Geometry: final body of the model. Coordinates: model frame, mm. A direction names the side the tool comes from. Round coordinates to 2 decimals unless told otherwise and drop trailing zeros. Write each loop counter-clockwise with the first axis right and the second up, starting at its lowest first coordinate (ties: lowest second). Pieces come first, ordered by that corner, then holes. Notation, with made-up numbers: (62.5, -7) -> (111.5, -7) arc R19 cw to (111.5, 4) -> close; hole circle Ø3 at (41.25, 0.25). An arc over 180 degrees is marked (long way). Use one line per item in the form item = value. Start each with the question number.
1. Cut plane D-D, the plane x = 1. Return the cut outline in (y, z), plus the area to 3 significant figures.
2. Pin query (flat end, axial travel): pin 1 Ø3.5 at (x, z) = (48, 0) entering from -Y; pin 2 Ø3 at (x, z) = (15, -0.5) entering from +Y; pin 3 Ø1 at (y, z) = (3.5, 1.5) entering from +X; pin 4 Ø1.5 at (y, z) = (3, 1) entering from -X. Return the tip coordinate at first contact, or that it passes through.
3. Reachability of faces 1 (the face through (20.974, 0.493, 0.672)), 2 (the face through (42, 7, -2)), 3 (the face through (36, 4, -3.1)) from +Z, -Z, +X, -X, +Y, -Y: full face, straight path, thin tool, end or side. Return the list, or none.
4. Cut plane B-B, the plane y = 7.5. State how many separate pieces and enclosed holes the cut face has, plus the area to 3 significant figures.
5. Cut plane A-A, the plane x = 24. Return the cut outline in (y, z).
6. Line query: L1, parallel to Z at x = 28, y = 5; L2, parallel to Y at x = 37.5, z = 1; L3, parallel to Z at x = 39, y = 5. Output: solid intervals per line, ascending.
```python
from build123d import *

# Parameters (mm, degrees)
BOSS_EXTRUDE1_DEPTH = 8
SKETCH5_R           = 3.1
CUT_EXTRUDE1_DEPTH  = 1
SKETCH6_R           = 2.4
CUT_EXTRUDE2_DEPTH  = 53.091266063
CUT_EXTRUDE3_START  = -1
SKETCH8_R           = 3.1
CUT_EXTRUDE3_DEPTH  = 1
LPATTERN3_COUNT     = 7
LPATTERN3_PITCH     = 8
CUT_EXTRUDE4_DEPTH  = 53.235045707
LPATTERN4_COUNT     = 6
LPATTERN4_PITCH     = 8


with BuildPart() as part:
    # Sketch3 → Boss-Extrude1 (new body)
    with BuildSketch(Plane(origin=(0, 0, 0), x_dir=(1, 0, 0), z_dir=(0, 1, 0))):
        with BuildLine():
            Line((0, 3.5), (48, 3.5))
            ThreePointArc((48, 3.5), (51.5, 0), (48, -3.5))
            Line((48, -3.5), (0, -3.5))
            ThreePointArc((0, -3.5), (-3.5, 0), (0, 3.5))
        make_face()
    extrude(amount=BOSS_EXTRUDE1_DEPTH)

    # Sketch5 → Cut-Extrude1 (cut)
    with BuildSketch(Plane(origin=(0, 0, 0), x_dir=(-1, 0, 0), z_dir=(0, -1, 0))):
        with Locations(Location((0, 0, 0), (0, 0, 90))):
            Circle(SKETCH5_R)
    cut_extrude1 = extrude(amount=-CUT_EXTRUDE1_DEPTH, mode=Mode.SUBTRACT)

    # Sketch6 → Cut-Extrude2 (cut, symmetric)
    with BuildSketch(Plane(origin=(0, 1, 0), x_dir=(-1, 0, 0), z_dir=(0, -1, 0))):
        with Locations(Location((0, 0, 0), (0, 0, 90))):
            Circle(SKETCH6_R)
    cut_extrude2 = extrude(amount=CUT_EXTRUDE2_DEPTH, both=True, mode=Mode.SUBTRACT)

    # Sketch8 → Cut-Extrude3 (cut)
    with BuildSketch(Plane(origin=(0, 8, 0), x_dir=(1, 0, 0), z_dir=(0, 1, 0)).offset(CUT_EXTRUDE3_START)):
        with Locations(Location((0, 0, 0), (0, 0, 90))):
            Circle(SKETCH8_R)
    cut_extrude3 = extrude(amount=CUT_EXTRUDE3_DEPTH, mode=Mode.SUBTRACT)

    # LPattern3: Cut-Extrude1, Cut-Extrude2, Cut-Extrude3 ×7
    with Locations(*[(i * LPATTERN3_PITCH, 0, 0) for i in range(1, LPATTERN3_COUNT)]):
        add(cut_extrude1, mode=Mode.SUBTRACT)
        add(cut_extrude2, mode=Mode.SUBTRACT)
        add(cut_extrude3, mode=Mode.SUBTRACT)

    # Sketch9 → Cut-Extrude4 (cut, symmetric)
    with BuildSketch(Plane(origin=(0, 8, 0), x_dir=(1, 0, 0), z_dir=(0, 1, 0))):
        with BuildLine():
            Line((2.814249456, 3.1), (5.185750544, 3.1))
            ThreePointArc((5.185750544, 3.1), (5.553697029, 2.856892908), (5.474391514, 2.423076923))
            ThreePointArc((5.474391514, 2.423076923), (4.5, 0), (5.474391514, -2.423076923))
            ThreePointArc((5.474391514, -2.423076923), (5.553697029, -2.856892908), (5.185750544, -3.1))
            Line((5.185750544, -3.1), (2.814249456, -3.1))
            ThreePointArc((2.814249456, -3.1), (2.446302971, -2.856892908), (2.525608486, -2.423076923))
            ThreePointArc((2.525608486, -2.423076923), (3.5, 0), (2.525608486, 2.423076923))
            ThreePointArc((2.525608486, 2.423076923), (2.446302971, 2.856892908), (2.814249456, 3.1))
        make_face()
    cut_extrude4 = extrude(amount=CUT_EXTRUDE4_DEPTH, both=True, mode=Mode.SUBTRACT)

    # LPattern4: Cut-Extrude4 ×6
    with Locations(*[(i * LPATTERN4_PITCH, 0, 0) for i in range(1, LPATTERN4_COUNT)]):
        add(cut_extrude4, mode=Mode.SUBTRACT)


solid = part.part
```
Outcome:
q1.outline = (0, -3.5) -> (8, -3.5) -> (8, -2.93) -> (7, -2.93) -> (7, -2.18) -> (1, -2.18) -> (1, -2.93) -> (0, -2.93) -> close; (0, 2.93) -> (1, 2.93) -> (1, 2.18) -> (7, 2.18) -> (7, 2.93) -> (8, 2.93) -> (8, 3.5) -> (0, 3.5) -> close
q1.area = 18.1 mm^2
q2.pin_1 = through
q2.pin_2 = 7
q2.pin_3 = 51.35
q2.pin_4 = -3.49
q3.face_1 = -Y
q3.face_2 = +Y
q3.face_3 = +Y, -Y
q4.separate_pieces = 1
q4.enclosed_holes = 13
q4.area = 91.7 mm^2
q5.outline = (0, -3.5) -> (8, -3.5) -> (8, -3.1) -> (7, -3.1) -> (7, -2.4) -> (1, -2.4) -> (1, -3.1) -> (0, -3.1) -> close; (0, 3.1) -> (1, 3.1) -> (1, 2.4) -> (7, 2.4) -> (7, 3.1) -> (8, 3.1) -> (8, 3.5) -> (0, 3.5) -> close
q6.L1 = -3.5 to -3.1, 3.1 to 3.5
q6.L2 = 1 to 7
q6.L3 = -3.5 to -2.18, 2.18 to 3.5
